```python
from build123d import *

# Parameters (mm, degrees)
F0_W            = 6.2
F0_H            = 6.2
F1_DEPTH        = 4.85
F3_DEPTH        = 1.53
F3_COPIES_COUNT = 4
F4_R            = 1.5
F5_DEPTH        = 0.92
F6_SIZE         = 0.2
F7_W            = 0.7
F7_H            = 3.5
F8_DEPTH        = 0.15


# Not quite as in the source:
# - a pattern or mirror of a feature is missing from the dataset's text; its kind, count and spacing are read off the source's solid


with BuildPart() as f1:
    # F0 (on Top) → F1 (new body)
    with BuildSketch(Plane.XY):
        Rectangle(F0_W, F0_H)
    extrude(amount=F1_DEPTH)

    # F2 (on face) → F3 (join)
    with BuildSketch(Plane.XY.offset(4.85)):
        with BuildLine():
            Line((1.2382979223, 2.8), (0, 2.8))
            Line((0, 2.8), (0, 0))
            Line((0, 0), (2.8, 0))
            Line((2.8, 0), (2.8, 1.4253550908))
            Line((2.8, 1.4253550908), (2.2382979223, 1.4253550908))
            ThreePointArc((2.2382979223, 1.4253550908), (1.5311911411, 1.7182483096), (1.2382979223, 2.4253550908))
            Line((1.2382979223, 2.4253550908), (1.2382979223, 2.8))
        make_face()
    f3 = extrude(amount=F3_DEPTH)

    # F3_copies: F3 ×4 about axis
    f3_copies_axis = Axis((0, 0, 0), (0, 0, 1))
    for i in range(1, F3_COPIES_COUNT):
        add(f3.rotate(f3_copies_axis, i * 360 / F3_COPIES_COUNT))

    # F4 (on face) → F5 (join)
    with BuildSketch(Plane.XY.offset(6.38)):
        Circle(F4_R)
    extrude(amount=F5_DEPTH)

    # F6
    f6_edges = [f1.edges().sort_by_distance(p)[0] for p in [
        (-1.5, 0, 7.3),
    ]]
    chamfer(f6_edges, length=F6_SIZE)

    # F7 (on Front) → F8 (join, symmetric)
    with BuildSketch(Plane.XZ):
        with Locations((-2.35, -1.75)):
            Rectangle(F7_W, F7_H)
    f8 = extrude(amount=F8_DEPTH, both=True)

    # F8_copies: F8 across plane
    add(f8.mirror(Plane(origin=(0, 0, 0), x_dir=(0, 0, 1), z_dir=(1, 0, 0))))


solid = f1.part
```
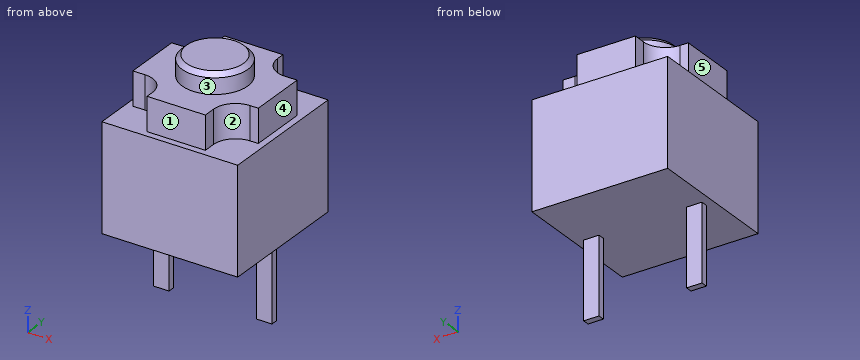
Work out the finished part from the listing and answer in its coordinate system (mm). Face numbers are marked on the shaded views. A direction names the side the tool comes from. Coordinates: 2 decimals unless noted, no trailing zeros. Loops run counter-clockwise (first coordinate to the right, second up) from the corner with the lowest first, then second, coordinate; pieces in that order, holes last.
1) Section D-D (y = -2) is taken. Give the vertices of the cut face in (x, z).
Results:
outline: (-3.1, 0) - (3.1, 0) - (3.1, 4.85) - (1.45, 4.85) - (1.45, 6.38) - (-1.33, 6.38) - (-1.33, 4.85) - (-3.1, 4.85) - close
2) Flat-ended cylindrical pins translate along their axes: pin 1 (0.8 mm diameter, centred on x = 2, z = -2, fed in from -Y); pin 2 (1 mm diameter, centred on x = -2, y = -0.5, fed in from -Z); pin 3 (1.2 mm diameter, centred on y = 0, z = 6, fed in from -X); pin 4 (0.6 mm diameter, centred on x = 2.5, z = -1.5, fed in from +Y). Find the tip coordinate at first contact, or state that the pin passes through.
Results:
pin 1: stops at y = -0.15
pin 2: stops at z = -3.5
pin 3: stops at x = -2.8
pin 4: stops at y = 0.15
3) For the marked faces 1, 2, 3, 4 and 5, determine the directions among +Z, -Z, +X, -X, +Y, -Y from which every point of the face is accessible in a straight line to the end or side of a thin tool.
Results:
face 1: +Z, +X, -X, -Y
face 2: +Z, +X, -Y
face 3: +Z
face 4: +Z, +X, +Y, -Y
face 5: +Z, -X, +Y, -Y
4) Section C-C (z = 6) is taken. Give the vertices of the cut face in (x, y).
Results:
outline: (-2.8, -1.43) - (-2.24, -1.43) arc R1 cw to (-1.24, -2.43) - (-1.24, -2.8) - (1.43, -2.8) - (1.43, -2.24) arc R1 cw to (2.43, -1.24) - (2.8, -1.24) - (2.8, 1.43) - (2.24, 1.43) arc R1 cw to (1.24, 2.43) - (1.24, 2.8) - (-1.43, 2.8) - (-1.43, 2.24) arc R1 cw to (-2.43, 1.24) - (-2.8, 1.24) - close
5) Section A-A (y = 0) is taken. Give the vertices of the cut face in (x, z), plus the area to 3 significant figures.
Results:
outline: (-3.1, 0) - (-2.7, 0) - (-2.7, -3.5) - (-2, -3.5) - (-2, 0) - (2, 0) - (2, -3.5) - (2.7, -3.5) - (2.7, 0) - (3.1, 0) - (3.1, 4.85) - (2.8, 4.85) - (2.8, 6.38) - (1.5, 6.38) - (1.5, 7.1) - (1.3, 7.3) - (-1.3, 7.3) - (-1.5, 7.1) - (-1.5, 6.38) - (-2.8, 6.38) - (-2.8, 4.85) - (-3.1, 4.85) - close
area: 46.3 mm2
6) Consider probe 1 along Z at (x, y) = (-1.75, 0.25); probe 2 along Z at (x, y) = (-1.5, 2.25); probe 3 along X at (y, z) = (0.25, 5). Determine where each line is inside the solid, lowest interval first.
Results:
probe 1: z = 0 to 6.38
probe 2: z = 0 to 4.85
probe 3: x = -2.8 to 2.8
7) Section B-B (x = 0) is taken. Give the vertices of the cut face in (y, z).
Results:
outline: (-3.1, 0) - (3.1, 0) - (3.1, 4.85) - (2.8, 4.85) - (2.8, 6.38) - (1.5, 6.38) - (1.5, 7.1) - (1.3, 7.3) - (-1.3, 7.3) - (-1.5, 7.1) - (-1.5, 6.38) - (-2.8, 6.38) - (-2.8, 4.85) - (-3.1, 4.85) - close
